```python
from build123d import *

# Parameters (mm, degrees)
BOSS_EXTRU_1_DEPTH      = 3
ESQUISSE2_W             = 20
ESQUISSE2_H             = 6
ENL_V_MAT_EXTRU_1_DEPTH = 10


with BuildPart() as part:
    # Esquisse1 → Boss.-Extru.1 (new body)
    with BuildSketch(Plane.XY):
        Polygon((-30, -45), (30, -45), (30, -29.5), (33, -29.5), (33, -15.5), (30, -15.5), (30, -7), (33, -7), (33, 7), (30, 7), (30, 15.5), (33, 15.5), (33, 29.5), (30, 29.5), (30, 45), (-30, 45), (-30, 29.5), (-33, 29.5), (-33, 15.5), (-30, 15.5), (-30, 7), (-33, 7), (-33, -7), (-30, -7), (-30, -15.5), (-33, -15.5), (-33, -29.5), (-30, -29.5), align=None)
    extrude(amount=BOSS_EXTRU_1_DEPTH)

    # Esquisse2 → Enlèv. mat.-Extru.1 (cut)
    with BuildSketch(Plane.XY.offset(3)):
        with Locations((0, 45)):
            Rectangle(ESQUISSE2_W, ESQUISSE2_H)
    extrude(amount=-ENL_V_MAT_EXTRU_1_DEPTH, mode=Mode.SUBTRACT)


solid = part.part
```
CAD build for the part. Positions are in the model's coordinates, mm. A direction names the side the tool comes from. Coordinates: 2 decimals unless noted, no trailing zeros. Loops run counter-clockwise (first coordinate to the right, second up) from the corner with the lowest first, then second, coordinate; pieces in that order, holes last. Notation, with made-up numbers: (22.5, 41.25) - (39.5, 41.25) arc R24 cw to (39.5, 61.25) - close; hole circle Ø2 at (47.5, 77). An arc over 180 degrees is marked (long way). Use CSV: the item, a comma, the result in double quotes. Start each with the question number.
Q1. Cut at C-C, the plane y = -13. List the corners of the cut face in (x, z).
Q2. Cut at B-B, the plane x = -3. List the corners of the cut face in (y, z), then the cut area to 3 significant figures.
Q3. 3-axis set-ups, long thin cutter, end or side, ignore diameter. For faces 5 (the flat face through (-31, 29.5, 1)), 6 (the flat face through (-31, 7, 1)), 7 (the flat face through (30, 37, 1)), 8 (the flat face through (31, 15.5, 1)): which of +Z, -Z, +X, -X, +Y, -Y reach the whole face in a straight line?
Q4. Probe probe 1 along X at (y, z) = (41, 1); probe 2 along Y at (x, z) = (-5, 0.8). List the from-to ranges inside material, lowest first. Write a range as from..to.
Q5. Two-plate mould, pull along X, no slides. Class faces 1 (the flat face through (33, 0, 1)), 2 (the flat face through (10, 43, 2)), 3 (the flat face through (-33, 0, 1)), 4 (the flat face through (32, -15.5, 1)): +X half, -X half, draft (parallel to the pull), parting line (faces both ways), or undercut.
Q6. Drop flat-ended pins along their axis: P1, Ø1.5, axis at y = 43.5, z = 1, coming from the -X side; P2, Ø1.5, axis at x = 31, z = 2, coming from the -Y side; P3, Ø0.9, axis at y = -40.5, z = 2, coming from the +X side. Give the stop position or say it passes through.
Here are the results:
1,outline,"(-30, 0) - (30, 0) - (30, 3) - (-30, 3) - close"
2,outline,"(-45, 0) - (42, 0) - (42, 3) - (-45, 3) - close"
2,area,"261 mm2"
3,face 5,"+Z, -Z, -X, +Y"
3,face 6,"+Z, -Z, -X"
3,face 7,"+Z, -Z, +X, +Y"
3,face 8,"+Z, -Z, +X"
4,probe 1,"-30..30"
4,probe 2,"-45..42"
5,face 1,"+X half"
5,face 2,"undercut"
5,face 3,"-X half"
5,face 4,"draft"
6,P1,"x = -30"
6,P2,"y = -29.5"
6,P3,"x = 30"
